Autodesk Inventor part; units mm, degrees
ref_plane "YZ Plane" through (0, 0, 0) normal (1, 0, 0) x (0, 1, 0)
ref_plane "XZ Plane" through (0, 0, 0) normal (0, 1, 0) x (-1, 0, 0)
ref_plane "XY Plane" through (0, 0, 0) normal (0, 0, 1) x (1, 0, 0)
sketch "Sketch1" plane through (0, 0, 0) normal (0, 1, 0) x (-1, 0, 0)
  line L0 (0, 0) -> (50, 0)
  line L1 (50, 0) -> (50, -22)
  line L2 (50, -22) -> (0, -22)
  line L3 (0, -22) -> (0, 0)
  dimension "d0" = 50
  dimension "d1" = 22
extrude "Extrusion1" add sketch "Sketch1" along normal blind 3
sketch "Sketch2" plane through (0, 0, 0) normal (0, -1, 0) x (1, 0, 0)
  line L0 (-50, 0) -> (0, 0)
  line L1 (0, -22) -> (-50, -22)
  line L2 (0, 0) -> (-3, 0)
  line L3 (-3, 0) -> (-3, -22)
  line L4 (-3, -22) -> (0, -22)
  line L5 (0, -22) -> (0, 0)
  dimension "d4" = 3
extrude "Extrusion2" add sketch "Sketch2" along normal blind 30
sketch "Sketch3" plane through (0, 3, 0) normal (0, 1, 0) x (1, 0, 0)
  circle A0 centre (-16.8, 11) radius 1.75
  line L0 (0, 22) -> (-50, 22)
  circle A1 centre (-42.2, 11) radius 1.75
  line L1 (-3, 0) -> (-29.8, 0)
  line L2 (-50, 0) -> (0, 0)
  line L3 (-29.8, 0) -> (-29.8, 11)
  circle A2 centre (-29.8, 11) radius 1.75
  dimension "d7" = 3.5
  dimension "d8" = 11
  dimension "d9" = 13.8
  dimension "d10" = 3.5
  dimension "d11" = 25.4
  dimension "d12" = 11
  dimension "d22" = 26.8
  dimension "d23" = 11
  dimension "d24" = 3.5
sketch "Sketch4" plane through (-3, 0, -22) normal (-1, 0, 0) x (0, 0, 1)
  line L0 (22, 0) -> (0, 0)
  line L1 (11, 0) -> (11, -11)
  circle A0 centre (11, -11) radius 1.75
  line L2 (11, -11) -> (11, -22)
  circle A1 centre (11, -22) radius 1.75
  dimension "d15" = 11
  dimension "d16" = 3.5
  dimension "d17" = 11
  dimension "d18" = 3.5
extrude "Extrusion4" cut sketch "Sketch4" against normal blind 3
fillet "Fillet1" radius 2 1 edges at (-3, 0, -11)
extrude "Extrusion5" cut sketch "Sketch3" against normal blind 3
properties part number "Right_BracketMount"
Could you check a few things on this model? Use its own coordinates, in mm. A direction names the side the tool comes from. Round coordinates to 2 decimals unless told otherwise and drop trailing zeros. Write each loop counter-clockwise with the first axis right and the second up, starting at its lowest first coordinate (ties: lowest second). Pieces come first, ordered by that corner, then holes. Notation, with made-up numbers: (-24, 21) - (6, 21) arc R31 cw to (6, 52) - close; hole circle Ø8 at (41.25, 22). An arc over 180 degrees is marked (long way). Use a Markdown table: item, result.
Q1. For faces 1 (the flat face through (-3, -16, -11)), 2 (the flat face through (-2, -30, -11)), which set-ups out of +Z, -Z, +X, -X, +Y, -Y let a thin tool reach every point of the face, with its end or its side?
Output values:
| item | result |
|---|---|
| face 1 | +Z, -Z, -X, -Y |
| face 2 | +Z, -Z, +X, -X, -Y |
Q2. Thinking about a two-plate mould opening in Z: for faces 3 (the cylindrical face through (-31.09, 1.52, -12.18)), 4 (the flat face through (-27, 0, -11)), 5 (the flat face through (-14, 1, -22)), which applies, released by +Z, released by -Z, zero draft, split by the parting line, or undercut?
Output values:
| item | result |
|---|---|
| face 3 | undercut |
| face 4 | zero draft |
| face 5 | released by -Z |
Q3. I want a section at D-D (z = -17.5). List the corners of the cut face in (x, y) for me, plus the area to 3 significant figures.
Output values:
| item | result |
|---|---|
| outline | (-50, 0) - (-5, 0) arc R2 cw to (-3, -2) - (-3, -30) - (0, -30) - (0, 3) - (-50, 3) - close |
| area | 241 mm2 |
Q4. I want a section at A-A (y = -22). List the corners of the cut face in (x, z) for me.
Output values:
| item | result |
|---|---|
| outline | (-3, -22) - (0, -22) - (0, -12.75) - (-3, -12.75) - close; (-3, -9.25) - (0, -9.25) - (0, 0) - (-3, 0) - close |
Q5. I want a section at C-C (x = -16.8). List the corners of the cut face in (y, z) for me.
Output values:
| item | result |
|---|---|
| outline | (0, -22) - (3, -22) - (3, -12.75) - (0, -12.75) - close; (0, -9.25) - (3, -9.25) - (3, 0) - (0, 0) - close |
Q6. For pin 1 (1.5 mm diameter, centred on y = -7, z = -4.5, fed in from -X); pin 2 (4 mm diameter, centred on x = -15, z = -13, fed in from -Y), each with a flat end and sliding along its axis, tell me the tip position at first contact or that it passes through.
Output values:
| item | result |
|---|---|
| pin 1 | x = -3 |
| pin 2 | y = 0 |
Q7. Please list where these lines run through material, in increasing order: L1, parallel to X at y = 1.65, z = -11; L2, parallel to Y at x = -2.3, z = -11; L3, parallel to Z at x = -29.8, y = 2.25.
Output values:
| item | result |
|---|---|
| L1 | -50 to -43.95, -40.45 to -31.55, -28.05 to -18.55, -15.05 to 0 |
| L2 | -30 to -23.75, -20.25 to -12.75, -9.25 to 3 |
| L3 | -22 to -12.75, -9.25 to 0 |
Q8. I want a section at B-B (z = -11). List the corners of the cut face in (x, y) for me.
Output values:
| item | result |
|---|---|
| outline | (-50, 0) - (-43.95, 0) - (-43.95, 3) - (-50, 3) - close; (-40.45, 0) - (-31.55, 0) - (-31.55, 3) - (-40.45, 3) - close; (-28.05, 0) - (-18.55, 0) - (-18.55, 3) - (-28.05, 3) - close; (-15.05, 0) - (-5, 0) arc R2 cw to (-3, -2) - (-3, -9.25) - (0, -9.25) - (0, 3) - (-15.05, 3) - close; (-3, -30) - (0, -30) - (0, -23.75) - (-3, -23.75) - close; (-3, -20.25) - (0, -20.25) - (0, -12.75) - (-3, -12.75) - close |
